```python
from build123d import *

# Parameters (mm, degrees)
BOSS_EXTRUDE1_DEPTH                             = 17.7
CSK_FOR_M3_FLAT_HEAD_MACHINE_SCREW1_D           = 3.6
CSK_FOR_M3_FLAT_HEAD_MACHINE_SCREW1_CSINK_D     = 6.3
CSK_FOR_M3_FLAT_HEAD_MACHINE_SCREW1_CSINK_ANGLE = 90
F_3_0MM_PRESS_DOWEL_HOLE1_D                     = 3


with BuildPart() as part:
    # Sketch1 → Boss-Extrude1 (new, symmetric)
    with BuildSketch(Plane(origin=(0, 0, 0), x_dir=(1, 0, 0), z_dir=(0, 1, 0))):
        Polygon((-14.5, 0), (14.5, 0), (14.5, 5), (19.5, 5), (19.5, 10), (-19.5, 10), (-19.5, 5), (-14.5, 5), align=None)
    extrude(amount=BOSS_EXTRUDE1_DEPTH, both=True)

    # CSK for M3 Flat Head Machine Screw1 (through all)
    with Locations(Plane(origin=(0, 0, -10), x_dir=(-1, 0, 0), z_dir=(0, 0, -1))):
        with Locations((0, 9.5), (-9.5, 0), (9.5, 0), (0, -9.5)):
            CounterSinkHole(CSK_FOR_M3_FLAT_HEAD_MACHINE_SCREW1_D / 2, CSK_FOR_M3_FLAT_HEAD_MACHINE_SCREW1_CSINK_D / 2, counter_sink_angle=CSK_FOR_M3_FLAT_HEAD_MACHINE_SCREW1_CSINK_ANGLE)

    # Ø3.0mm Press Dowel Hole1 (through all)
    with Locations(Plane(origin=(-4.77392109, 17.7, -4.32762779), x_dir=(0, 0, 1), z_dir=(0, 1, 0))):
        with Locations((0, 0), (0, 9.54784218)):
            Hole(F_3_0MM_PRESS_DOWEL_HOLE1_D / 2)


solid = part.part
```
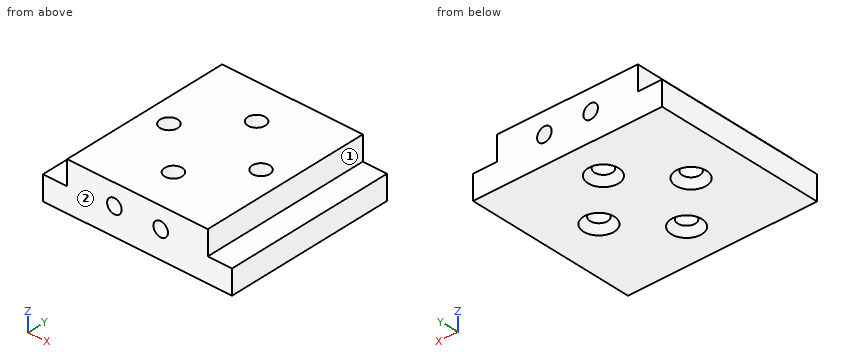
Part model, mm, in its own coordinate system. Face numbers are marked on the shaded views. A direction names the side the tool comes from. Coordinates: 2 decimals unless noted, no trailing zeros. Order: outer loops, then holes, each group sorted by start corner. A loop starts at its lowest first (then second) coordinate and runs counter-clockwise, first axis right, second up. Notation, with made-up numbers: (2, -21.75) - (35, -21.75) arc R26 cw to (35, 17.25) - close; hole circle Ø4 at (-2.5, 52). An arc over 180 degrees is marked (long way). Return JSON: item names as keys, results as strings. Group by question number.
Item 1: Which spindle directions (+Z, -Z, +X, -X, +Y, -Y) get a long thin tool onto all of the face, cutting with end or side? Do the marked faces 1 and 2. Say none if no direction does.
Item 2: Cut at D-D (z = -8). List the corners of the cut face in (x, y).
Item 3: Cut at C-C (x = -9.5). List the corners of the cut face in (y, z), plus the area to 3 significant figures.
Item 4: Cut at A-A (x = 0). List the corners of the cut face in (y, z).
Item 5: Drill centre lines: probe 1 along X at (y, z) = (0, -6); probe 2 along X at (y, z) = (0, -2.5); probe 3 along Y at (x, z) = (0, -4.5). Where is each one in solid material? Low to high. Write a range as from..to.
Item 6: Cut at B-B (y = 9.5). List the corners of the cut face in (x, z).
Item 7: Pin check, flat tips, straight feed: pin 1 (4.5 mm diameter, centred on x = 0, y = 9.5, fed in from -Z); pin 2 (4 mm diameter, centred on x = 9.5, y = 0, fed in from -Z); pin 3 (2.5 mm diameter, centred on y = -2, z = -3, fed in from -X). Stop position of each tip, or through.
Check values:
{
 "1": {"face 1": "+Z, +X, +Y, -Y", "face 2": "+Z, -Z, +X, -X, -Y"},
 "2": {"outline": "(-19.5, -17.7) - (19.5, -17.7) - (19.5, 17.7) - (-19.5, 17.7) - close; hole circle Ø3.6 at (-9.5, 0); hole circle Ø3.6 at (0, -9.5); hole circle Ø3.6 at (0, 9.5); hole circle Ø3.6 at (9.5, 0)"},
 "3": {"outline": "(-17.7, -10) - (-3.15, -10) - (-1.8, -8.65) - (-1.8, 0) - (-17.7, 0) - close; (1.8, -8.65) - (3.15, -10) - (17.7, -10) - (17.7, 0) - (1.8, 0) - close", "area": "316 mm2"},
 "4": {"outline": "(-17.7, -10) - (-12.65, -10) - (-11.3, -8.65) - (-11.3, 0) - (-17.7, 0) - close; (-7.7, -8.65) - (-6.35, -10) - (6.35, -10) - (7.7, -8.65) - (7.7, 0) - (-7.7, 0) - close; (11.3, -8.65) - (12.65, -10) - (17.7, -10) - (17.7, 0) - (11.3, 0) - close"},
 "5": {"probe 1": "x = -19.5..-11.3, -7.7..7.7, 11.3..19.5", "probe 2": "x = -14.5..-11.3, -7.7..7.7, 11.3..14.5", "probe 3": "y = -17.7..-11.3, -7.7..7.7, 11.3..17.7"},
 "6": {"outline": "(-19.5, -10) - (-3.15, -10) - (-1.8, -8.65) - (-1.8, 0) - (-14.5, 0) - (-14.5, -5) - (-19.5, -5) - close; (1.8, -8.65) - (3.15, -10) - (19.5, -10) - (19.5, -5) - (14.5, -5) - (14.5, 0) - (1.8, 0) - close; hole circle Ø3 at (-4.77, -4.33); hole circle Ø3 at (4.77, -4.33)"},
 "7": {"pin 1": "stops at z = -9.1", "pin 2": "stops at z = -8.85", "pin 3": "stops at x = -14.5"}
}
